```python
from build123d import *

# Parameters (mm, degrees)
MODEL_R                 = 1.5
SALIENTE_EXTRUIR1_DEPTH = 3


with BuildPart() as part:
    # Model → Saliente-Extruir1 (new body)
    with BuildSketch(Plane.XY):
        with BuildLine():
            Line((421.555570316, 186.576624848), (448.555570316, 168.576624848))
            ThreePointArc((448.555570316, 168.576624848), (449.399739312, 168.320548983), (450.277645761, 168.234082745))
            Line((450.277645761, 168.234082745), (459.277645761, 168.234082745))
            ThreePointArc((459.277645761, 168.234082745), (463.777645761, 172.734082745), (459.277645761, 177.234082745))
            Line((459.277645761, 177.234082745), (452.141606792, 177.234082745))
            Line((452.141606792, 177.234082745), (445.777645761, 183.598043775))
            Line((445.777645761, 183.598043775), (445.777645761, 190.734082745))
            ThreePointArc((445.777645761, 190.734082745), (444.459626276, 193.91606326), (441.277645761, 195.234082745))
            Line((441.277645761, 195.234082745), (425.141606792, 195.234082745))
            Line((425.141606792, 195.234082745), (417.459626276, 202.91606326))
            ThreePointArc((417.459626276, 202.91606326), (411.095665246, 202.91606326), (411.095665246, 196.552102229))
            Line((411.095665246, 196.552102229), (420.095665246, 187.552102229))
            ThreePointArc((420.095665246, 187.552102229), (420.777579713, 186.992469489), (421.555570316, 186.576624848))
        make_face()
        with Locations((441.277645761, 190.734082745)):
            Circle(MODEL_R, mode=Mode.SUBTRACT)
        with Locations((459.277645761, 172.734082745)):
            Circle(MODEL_R, mode=Mode.SUBTRACT)
        with Locations((423.277645761, 190.734082745)):
            Circle(MODEL_R, mode=Mode.SUBTRACT)
        with Locations((432.277645761, 190.734082745)):
            Circle(MODEL_R, mode=Mode.SUBTRACT)
        with Locations((414.277645761, 199.734082745)):
            Circle(MODEL_R, mode=Mode.SUBTRACT)
        with Locations((441.277645761, 181.734082745)):
            Circle(MODEL_R, mode=Mode.SUBTRACT)
        with Locations((436.777645761, 186.234082745)):
            Circle(MODEL_R, mode=Mode.SUBTRACT)
        with Locations((445.777645761, 177.234082745)):
            Circle(MODEL_R, mode=Mode.SUBTRACT)
    extrude(amount=SALIENTE_EXTRUIR1_DEPTH)


solid = part.part
```
The listing builds one solid part. Answer for the finished solid, in the listing's coordinates (mm). A direction names the side the tool comes from. Round coordinates to 2 decimals unless told otherwise and drop trailing zeros. Order: outer loops, then holes, each group sorted by start corner. A loop starts at its lowest first (then second) coordinate and runs counter-clockwise, first axis right, second up. Notation, with made-up numbers: (-18.75, 21.5) -> (36.25, 21.5) arc R19 cw to (36.25, 54.5) -> close; hole circle Ø11 at (-28.75, 21.5). An arc over 180 degrees is marked (long way). Answer as CSV lines item,"result".
Q1. For a pull along Y with two mould halves and no side action, classify faces 1 (the cylindrical face through (411.17, 202.99, 1.48)), 2 (the flat face through (433, 195.234, 1)), 3 (the cylindrical face through (457.78, 172.8, 1.48)), 4 (the cylindrical face through (440.95, 180.27, 1.48)) as +Y half, -Y half, draft (parallel to the pull), parting line (faces both ways), or undercut.
Computed values:
face 1,"parting line"
face 2,"+Y half"
face 3,"undercut"
face 4,"undercut"
Q2. Given pin 1 (1 mm diameter, centred on y = 174.5, z = 2, fed in from +X); pin 2 (1.5 mm diameter, centred on x = 432, z = 1, fed in from +Y), each flat-ended and moving along its own axis, determine where each tip first touches the part or whether it passes through.
Computed values:
pin 1,"stops at x = 463.6"
pin 2,"stops at y = 195.23"
Q3. Which of the six approach directions +Z, -Z, +X, -X, +Y, -Y give full straight-line access (tool end or side, diameter ignored) to faces 5 (the flat face through (456, 177.234, 1)), 6 (the flat face through (415.53, 192.12, 1.48))?
Computed values:
face 5,"+Z, -Z, +X, +Y"
face 6,"+Z, -Z, -X, -Y"
Q4. Consider line 1 (X direction, y = 190, z = 2.35); line 2 (Y direction, x = 442.5, z = 2.15); line 3 (Y direction, x = 441, z = 2.6). Determine where each line is inside the solid, lowest interval first. Write a range as from..to.
Computed values:
line 1,"x = 417.65..421.97, 424.59..430.97, 433.59..439.97, 442.59..445.78"
line 2,"y = 172.61..180.86, 182.6..189.86, 191.6..195.06"
line 3,"y = 173.61..180.26, 183.21..189.26, 192.21..195.23"
Q5. A cutting plane is placed at B-B on z = 1.6. Give the number of separate pieces and of enclosed holes in the cut face, plus the area to 3 significant figures.
Computed values:
separate pieces,"1"
enclosed holes,"8"
area,"645 mm^2"
Q6. A cutting plane is placed at A-A on x = 446.5. Determine the outline of the cut face in (y, z), plus the area to 3 significant figures.
Computed values:
outline,"(169.95, 0) -> (175.92, 0) -> (175.92, 3) -> (169.95, 3) -> close; (178.55, 0) -> (182.88, 0) -> (182.88, 3) -> (178.55, 3) -> close"
area,"30.9 mm^2"
Q7. A cutting plane is placed at D-D on x = 456.5. Determine the outline of the cut face in (y, z), plus the area to 3 significant figures.
Computed values:
outline,"(168.23, 0) -> (177.23, 0) -> (177.23, 3) -> (168.23, 3) -> close"
area,"27.0 mm^2"
Q8. A cutting plane is placed at C-C on y = 178. Determine the outline of the cut face in (x, z).
Computed values:
outline,"(434.42, 0) -> (444.49, 0) -> (444.49, 3) -> (434.42, 3) -> close; (447.07, 0) -> (451.38, 0) -> (451.38, 3) -> (447.07, 3) -> close"
